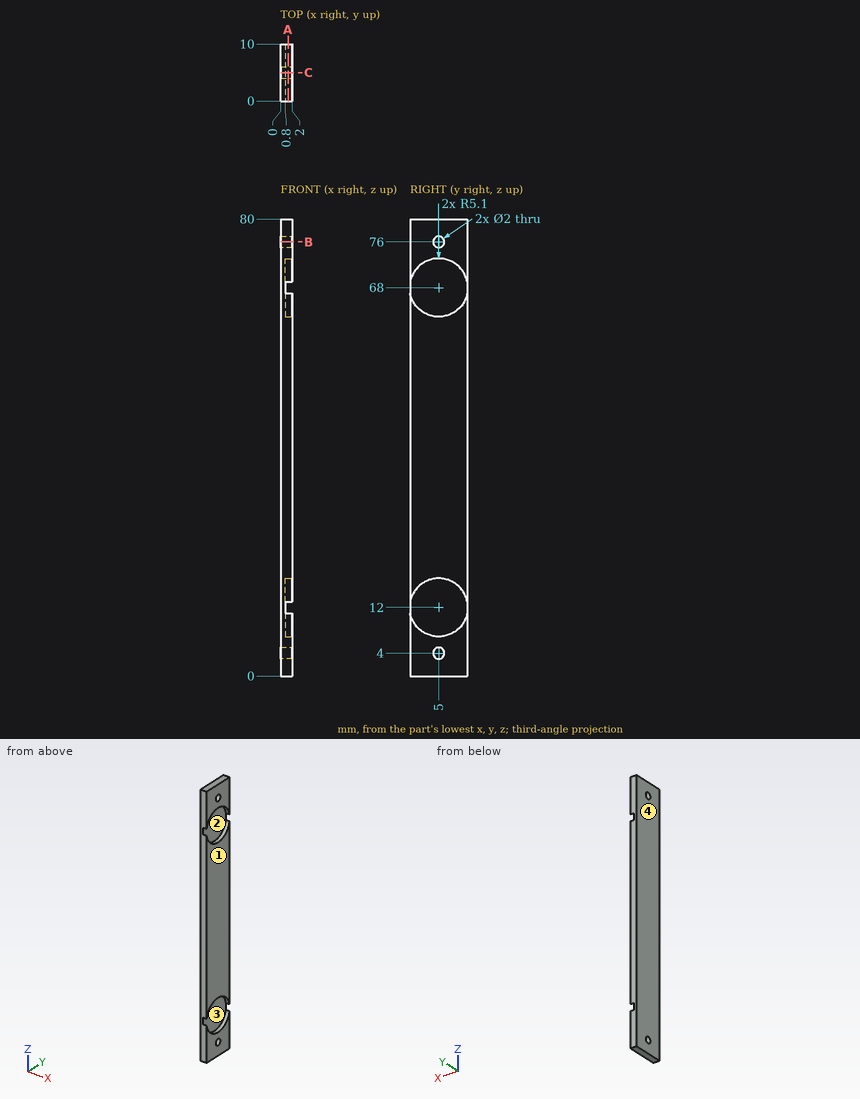
Input: dimensioned drawing with shaded views. Units: mm. Origin: part minimum x, y, z. A direction names the side the tool comes from. Coordinates: 2 decimals unless noted, no trailing zeros. Order: outer loops, then holes, each group sorted by start corner. A loop starts at its lowest first (then second) coordinate and runs counter-clockwise, first axis right, second up. Notation, with made-up numbers: (-19, 76) -> (12, 76) arc R28 cw to (12, 106) -> close; hole circle Ø1 at (39.25, -13). An arc over 180 degrees is marked (long way). Use CSV: the item, a comma, the result in double quotes.
1) Line query: line 1 (Z direction, x = 1.9, y = 1.25); line 2 (Z direction, x = 1.75, y = 3.75); line 3 (Y direction, x = 0.5, z = 76). Output: solid intervals per line, ascending.
Findings:
line 1,"z = 0 to 8.54, 15.46 to 64.54, 71.46 to 80"
line 2,"z = 0 to 7.06, 16.94 to 63.06, 72.94 to 80"
line 3,"y = 0 to 4, 6 to 10"
2) Mould query, pull axis Y, two halves, no side actions, for the marked faces 3 and 4. Classes: +Y half, -Y half, draft (parallel to the pull), parting line (faces both ways), or undercut.
Findings:
face 3,"undercut"
face 4,"draft"
3) Section B-B on z = 76. Output: boundary loops of the cut face in (x, y), then the cut area to 3 significant figures.
Findings:
outline,"(0, 0) -> (2, 0) -> (2, 4) -> (0, 4) -> close; (0, 6) -> (2, 6) -> (2, 10) -> (0, 10) -> close"
area,"16.0 mm^2"
4) Section A-A on x = 1.3. Output: boundary loops of the cut face in (y, z), then the cut area to 3 significant figures.
Findings:
outline,"(0, 0) -> (10, 0) -> (10, 11) arc R5.1 cw to (0, 11) -> close; (0, 13) arc R5.1 cw to (10, 13) -> (10, 67) arc R5.1 cw to (0, 67) -> close; (0, 69) arc R5.1 cw to (10, 69) -> (10, 80) -> (0, 80) -> close; hole circle Ø2 at (5, 4); hole circle Ø2 at (5, 76)"
area,"631 mm^2"
5) Access query for the marked faces 1 and 2. Directions: +Z, -Z, +X, -X, +Y, -Y. A direction counts if a zero-diameter tool reaches every point of the face in a straight line with its end or side. Return the directions, or none.
Findings:
face 1,"+Z, -Z, +X, +Y, -Y"
face 2,"+X"
6) Pin query (flat end, axial travel): pin 1 Ø2 at (y, z) = (8.5, 68.5) entering from +X. Return the tip coordinate at first contact, or that it passes through.
Findings:
pin 1,"stops at x = 0.8"
7) Section C-C on y = 5. Output: boundary loops of the cut face in (x, z), then the cut area to 3 significant figures.
Findings:
outline,"(0, 0) -> (2, 0) -> (2, 3) -> (0, 3) -> close; (0, 5) -> (2, 5) -> (2, 6.9) -> (0.8, 6.9) -> (0.8, 17.1) -> (2, 17.1) -> (2, 62.9) -> (0.8, 62.9) -> (0.8, 73.1) -> (2, 73.1) -> (2, 75) -> (0, 75) -> close; (0, 77) -> (2, 77) -> (2, 80) -> (0, 80) -> close"
area,"128 mm^2"
